```python
from build123d import *

# Parameters (mm, degrees)
SKETCH1_R           = 2.1
BOSS_EXTRUDE1_DEPTH = 15.5
SKETCH2_R           = 14
CUT_EXTRUDE1_DEPTH  = 16.5
CUT_EXTRUDE2_START  = -18
SKETCH4_R           = 3
CUT_EXTRUDE2_DEPTH  = 4.325206
CIRPATTERN1_COUNT   = 3


with BuildPart() as part:
    # Sketch1 → Boss-Extrude1 (new body)
    with BuildSketch(Plane(origin=(0, 0, 0), x_dir=(1, 0, 0), z_dir=(0, 1, 0))):
        with BuildLine():
            Line((-4, -17.549928775), (-4, -22))
            ThreePointArc((-4, -22), (0, -26), (4, -22))
            Line((4, -22), (4, -17.549928775))
            ThreePointArc((4, -17.549928775), (15.588457268, -9), (17.198684154, 5.310862772))
            Line((17.198684154, 5.310862772), (21.052558883, 7.535898385))
            ThreePointArc((21.052558883, 7.535898385), (22.516660498, 13), (17.052558883, 14.464101615))
            Line((17.052558883, 14.464101615), (13.198684154, 12.239066003))
            ThreePointArc((13.198684154, 12.239066003), (0, 18), (-13.198684154, 12.239066003))
            Line((-13.198684154, 12.239066003), (-17.052558883, 14.464101615))
            ThreePointArc((-17.052558883, 14.464101615), (-22.516660498, 13), (-21.052558883, 7.535898385))
            Line((-21.052558883, 7.535898385), (-17.198684154, 5.310862772))
            ThreePointArc((-17.198684154, 5.310862772), (-15.588457268, -9), (-4, -17.549928775))
        make_face()
        with Locations((0, -22)):
            Circle(SKETCH1_R, mode=Mode.SUBTRACT)
        with Locations((-19.052558883, 11)):
            Circle(SKETCH1_R, mode=Mode.SUBTRACT)
        with Locations((19.052558883, 11)):
            Circle(SKETCH1_R, mode=Mode.SUBTRACT)
    extrude(amount=BOSS_EXTRUDE1_DEPTH)

    # Sketch2 → Cut-Extrude1 (cut, through all)
    with BuildSketch(Plane(origin=(0, 15.5, 0), x_dir=(1, 0, 0), z_dir=(0, 1, 0))):
        Circle(SKETCH2_R)
    extrude(amount=-CUT_EXTRUDE1_DEPTH, mode=Mode.SUBTRACT)

    # Sketch3 → Revolve1 (revolve)
    with BuildSketch(Plane.XY):
        Polygon((14, 10), (12.058684154, 7.5), (12.058684154, 3.5), (13.198684154, 3.5), (13.198684154, 0), (14, 0), (14.499168446, 0), (14.499168446, 10), align=None)
    revolve(axis=Axis((0, 0, 0), (0, 1, 0)))

    # Sketch4 → Cut-Extrude2 (cut)
    with BuildSketch(Plane.XY.offset(CUT_EXTRUDE2_START)):
        with Locations((0, 15.5)):
            Circle(SKETCH4_R)
    cut_extrude2 = extrude(amount=CUT_EXTRUDE2_DEPTH, mode=Mode.SUBTRACT)

    # CirPattern1: Cut-Extrude2 ×3 about axis
    cirpattern1_axis = Axis((0, 0, 0), (0, 1, 0))
    for i in range(1, CIRPATTERN1_COUNT):
        add(cut_extrude2.rotate(cirpattern1_axis, i * 360 / CIRPATTERN1_COUNT), mode=Mode.SUBTRACT)


solid = part.part
```
CAD build for the part. Positions are in the model's coordinates, mm. A direction names the side the tool comes from. Give positions to 0.01 mm unless a question says otherwise; leave off trailing zeros. Loops run counter-clockwise (first coordinate to the right, second up) from the corner with the lowest first, then second, coordinate; pieces in that order, holes last. Notation, with made-up numbers: (45, 39.25) - (59, 39.25) arc R34 cw to (59, 73.25) - close; hole circle Ø4 at (-34.75, 56.5). An arc over 180 degrees is marked (long way). Put each result on its own line as item: value.
Q1. Slice it at D-D (y = 11.5). Give the cut face in (x, z), plus the area to 3 significant figures.
Filled in:
outline: (-21.05, -7.54) arc R4 ccw to (-17.05, -14.46) - (-13.2, -12.24) arc R18 ccw to (13.2, -12.24) - (17.05, -14.46) arc R4 ccw to (21.05, -7.54) - (17.2, -5.31) arc R18 ccw to (4, 17.55) - (4, 22) arc R4 ccw to (-4, 22) - (-4, 17.55) arc R18 ccw to (-17.2, -5.31) - close; hole circle Ø4.2 at (-19.05, -11); hole circle Ø28 at (0, 0); hole circle Ø4.2 at (0, 22); hole circle Ø4.2 at (19.05, -11)
area: 536 mm²
Q2. Tool access for faces 1 (the face through (19.1, 7.64, -6.41)), 2 (the face through (-19.153, 7.642, -6.439)), 3 (the face through (-6, 3.5, 11)), 4 (the face through (4, 8, 20)), 5 (the face through (15.153, 7.642, -13.367)): list every direction of +Z, -Z, +X, -X, +Y, -Y with a clear straight run to the whole face (end or side of a thin tool).
Filled in:
face 1: +X, +Y, -Y
face 2: -X, +Y, -Y
face 3: -Y
face 4: +Z, +X, +Y, -Y
face 5: -Z, +Y, -Y
Q3. Mould opens along X. For faces 6 (the face through (1.13, 7.64, 20.23)), 7 (the face through (-5.2, 0, -12.4)), 8 (the face through (-4, 8, 20)) say: pulls with the +X half, pulls with the -X half, needs draft (parallel to the pull), parting line crosses it, or undercut.
Filled in:
face 6: undercut
face 7: needs draft
face 8: pulls with the -X half
Q4. Slice it at C-C (z = -10). Give the number of separate pieces and of enclosed holes in the cut face, plus the area to 3 significant figures.
Filled in:
separate pieces: 4
enclosed holes: 0
area: 333 mm²
Q5. Slice it at A-A (x = 0). Give the cut face in (y, z), plus the area to 3 significant figures.
Filled in:
outline: (0, -18) - (12.5, -18) - (12.5, -14) - (10, -14) - (7.5, -12.06) - (3.5, -12.06) - (3.5, -13.2) - (0, -13.2) - close; (0, 13.2) - (3.5, 13.2) - (3.5, 12.06) - (7.5, 12.06) - (10, 14) - (15.5, 14) - (15.5, 19.9) - (0, 19.9) - close; (0, 24.1) - (15.5, 24.1) - (15.5, 26) - (0, 26) - close
area: 197 mm²
Q6. Flat gauge pins, fed straight in: pin 1 (1 mm diameter, centred on x = 7, y = 9.5, fed in from -Z); pin 2 (2 mm diameter, centred on y = 6, z = 4, fed in from -X); pin 3 (5 mm diameter, centred on y = 10, z = 19, fed in from +X). Where does each tip first touch, or does it go through?
Filled in:
pin 1: stops at z = -16.79
pin 2: stops at x = -17.75
pin 3: stops at x = 7.19
Q7. Probe line 1 along Z through (x, y) = (0, 5.45); line 2 along Z through (x, y) = (0, 12.4); line 3 along Z through (x, y) = (0, 13.8). List the from-to ranges inside material, lowest first.
Filled in:
line 1: z = -18 to -12.06, 12.06 to 19.9, 24.1 to 26
line 2: z = -18 to -14, 14 to 19.9, 24.1 to 26
line 3: z = 14 to 19.9, 24.1 to 26
Q8. Slice it at B-B (y = 1.75). Give the cut face in (x, z).
Filled in:
outline: (-21.05, -7.54) arc R4 ccw to (-17.05, -14.46) - (-13.2, -12.24) arc R18 ccw to (13.2, -12.24) - (17.05, -14.46) arc R4 ccw to (21.05, -7.54) - (17.2, -5.31) arc R18 ccw to (4, 17.55) - (4, 22) arc R4 ccw to (-4, 22) - (-4, 17.55) arc R18 ccw to (-17.2, -5.31) - close; hole circle Ø4.2 at (-19.05, -11); hole circle Ø26.4 at (0, 0); hole circle Ø4.2 at (0, 22); hole circle Ø4.2 at (19.05, -11)
